from build123d import *

# Parameters (mm, degrees)
F0_R            = 41.5
F1_DEPTH        = 25
F3_D            = 12.6
F3_COPIES_COUNT = 6
F4_R            = 17.5
F5_DEPTH        = 25.001


# Not quite as in the source:
# - a pattern or mirror of a feature is missing from the dataset's text; its kind, count and spacing are read off the source's solid


with BuildPart() as f1:
    # F0 (on Top) → F1 (new body)
    with BuildSketch(Plane.XY):
        Circle(F0_R)
    extrude(amount=F1_DEPTH)

    # F3 (through all)
    with Locations(Plane.XY.offset(25)):
        with Locations((0, 32.5)):
            f3 = Hole(F3_D / 2)

    # F3_copies: F3 ×6 about axis
    f3_copies_axis = Axis((0, 0, 0), (0, 0, 1))
    for i in range(1, F3_COPIES_COUNT):
        add(f3.rotate(f3_copies_axis, i * 360 / F3_COPIES_COUNT), mode=Mode.SUBTRACT)

    # F4 (on face) → F5 (cut, through all)
    with BuildSketch(Plane.XY.offset(25)):
        Circle(F4_R)
    extrude(amount=-F5_DEPTH, mode=Mode.SUBTRACT)


solid = f1.part
Could you check a few things on this model? Use its own coordinates, in mm. Round coordinates to 2 decimals unless told otherwise and drop trailing zeros. Order: outer loops, then holes, each group sorted by start corner. A loop starts at its lowest first (then second) coordinate and runs counter-clockwise, first axis right, second up.
(1) Please list where these lines run through material, in increasing order: line 1 along Y through (x, z) = (0, 19); line 2 along Y through (x, z) = (-33.5, 15.75); line 3 along X through (y, z) = (18, 16.5).
Response values:
line 1: y = -41.5 to -38.8, -26.2 to -17.5, 17.5 to 26.2, 38.8 to 41.5
line 2: y = -24.49 to -19.57, -12.93 to 12.93, 19.57 to 24.49
line 3: x = -37.39 to -34.2, -22.09 to 22.09, 34.2 to 37.39
(2) Imagine slicing it at A-A (x = 0). Write out the boundary of the cut face in (y, z), plus the area to 3 significant figures.
Response values:
outline: (-41.5, 0) - (-38.8, 0) - (-38.8, 25) - (-41.5, 25) - close; (-26.2, 0) - (-17.5, 0) - (-17.5, 25) - (-26.2, 25) - close; (17.5, 0) - (26.2, 0) - (26.2, 25) - (17.5, 25) - close; (38.8, 0) - (41.5, 0) - (41.5, 25) - (38.8, 25) - close
area: 570 mm2
(3) I'm going to push flat-ended pins straight in: pin 1 (5 mm diameter, centred on y = 23, z = 11.5, fed in from +X); pin 2 (7.5 mm diameter, centred on x = 0, y = -32.5, fed in from +Z); pin 3 (1 mm diameter, centred on y = -17, z = 17.5, fed in from -X); pin 4 (2 mm diameter, centred on x = 21, z = 9, fed in from -Y). Where does each tip first touch, or does it pass through?
Response values:
pin 1: stops at x = 36.08
pin 2: passes through
pin 3: stops at x = -38.08
pin 4: stops at y = -36.36
(4) Imagine slicing it at C-C (y = 20.5). Write out the boundary of the cut face in (x, z).
Response values:
outline: (-36.08, 0) - (-32.8, 0) - (-32.8, 25) - (-36.08, 25) - close; (-23.5, 0) - (23.5, 0) - (23.5, 25) - (-23.5, 25) - close; (32.8, 0) - (36.08, 0) - (36.08, 25) - (32.8, 25) - close
(5) Imagine slicing it at B-B (y = 0). Write out the boundary of the cut face in (x, z), plus the area to 3 significant figures.
Response values:
outline: (-41.5, 0) - (-17.5, 0) - (-17.5, 25) - (-41.5, 25) - close; (17.5, 0) - (41.5, 0) - (41.5, 25) - (17.5, 25) - close
area: 1,200 mm2
(6) If we mould it in two halves opening along X, with no side actions, what happens to faces 1 (the flat face through (-1, -18, 25)), 2 (the cylindrical face through (39.584, 12.465, 12.325)), 3 (the cylindrical face through (-33.965, -18.663, 12.325))? For each: released by +X, released by -X, zero draft, split by the parting line, or undercut.
Response values:
face 1: zero draft
face 2: split by the parting line
face 3: undercut
(7) Imagine slicing it at D-D (y = -14). Write out the boundary of the cut face in (x, z).
Response values:
outline: (-39.07, 0) - (-34.03, 0) - (-34.03, 25) - (-39.07, 25) - close; (-22.26, 0) - (-10.5, 0) - (-10.5, 25) - (-22.26, 25) - close; (10.5, 0) - (22.26, 0) - (22.26, 25) - (10.5, 25) - close; (34.03, 0) - (39.07, 0) - (39.07, 25) - (34.03, 25) - close
